from build123d import *

# Parameters (mm, degrees)
SKETCH_2_W          = 16
SKETCH_2_H          = 35
EXTRUDE_1_DEPTH     = 2
EXTRUDE_START       = 1.5
SKETCH_4_R          = 2.6
EXTRUDE_2_DEPTH     = 3
FILLET_2_R          = 1.5
SKETCH_5_R          = 2.1
CUT_EXTRUDE_1_DEPTH = 33.345787979


with BuildPart() as part:
    # 草圖2 → 填料-伸長1 (new body)
    with BuildSketch(Plane(origin=(0, 0, 0), x_dir=(1, 0, 0), z_dir=(0, 1, 0))):
        Rectangle(SKETCH_2_W, SKETCH_2_H)
    extrude(amount=EXTRUDE_1_DEPTH)

    # 草圖4 → 填料-伸長2 (add)
    with BuildSketch(Plane.XY.offset(EXTRUDE_START)):
        with BuildLine():
            Line((8, 20), (8, 2))
            Line((8, 2), (-8, 2))
            Line((-8, 2), (-8, 20))
            ThreePointArc((-8, 20), (0, 28), (8, 20))
        make_face()
        with Locations((0, 20)):
            Circle(SKETCH_4_R, mode=Mode.SUBTRACT)
    extrude_2 = extrude(amount=EXTRUDE_2_DEPTH)

    # 鏡射1: 填料-伸長2 across plane
    add(extrude_2.mirror(Plane.XY))

    # 圓角2
    fillet_2_edges = [part.edges().sort_by_distance(p)[0] for p in [
        (0, 2, 4.5),
        (0, 2, 1.5),
        (0, 2, -4.5),
        (0, 2, -1.5),
    ]]
    fillet(fillet_2_edges, radius=FILLET_2_R - 0.0001)  # a hair under: the kernel refuses the full size

    # 草圖5 → 除料-伸長1 (cut, through all)
    with BuildSketch(Plane(origin=(0, 2, 0), x_dir=(1, 0, 0), z_dir=(0, 1, 0))):
        with Locations(Location((0, -12.5, 0), (0, 0, 270))):
            Circle(SKETCH_5_R)
        with Locations(Location((0, 12.5, 0), (0, 0, 90))):
            Circle(SKETCH_5_R)
    extrude(amount=-CUT_EXTRUDE_1_DEPTH, mode=Mode.SUBTRACT)


solid = part.part
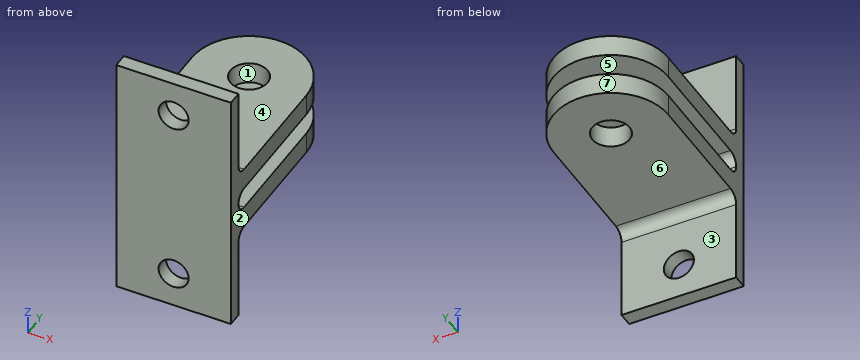
Read the model definition and answer for the solid it produces. Units are mm, in the model's axes. Face numbers are marked on the shaded views. A direction names the side the tool comes from. Coordinates: 2 decimals unless noted, no trailing zeros. Loops run counter-clockwise (first coordinate to the right, second up) from the corner with the lowest first, then second, coordinate; pieces in that order, holes last.
Q1. The part is cut by section B-B on y = 8. Write down the section's boundary in (x, z), and give its area (3 significant figures).
Q2. The part is cut by section C-C on z = -12.5. Write down the section's boundary in (x, y), and give its area (3 significant figures).
Q3. The mould has two halves that part along X. Classify the marked faces 1, 2 and 3: +X half, -X half, draft (parallel to the pull), parting line (faces both ways), or undercut.
Q4. Consider probe 1 along Y at (x, z) = (0, -3.2); probe 2 along Z at (x, y) = (-3, 14.5); probe 3 along X at (y, z) = (0.4, 12.5). Determine where each line is inside the solid, lowest interval first.
Q5. The part is cut by section A-A on x = 0. Give the number of separate pieces and of enclosed holes in the cut face, and give its area (3 significant figures).
Q6. The part is cut by section D-D on y = 21.25. Write down the section's boundary in (x, z).
Q7. Which of the six approach directions +Z, -Z, +X, -X, +Y, -Y give full straight-line access (tool end or side, diameter ignored) to the marked faces 4, 5, 6 and 7?
Q8. Each of these flat-tipped pins is pushed along its axis until it touches: pin 1 Ø3.5 at (x, z) = (3, 14.5) entering from +Y; pin 2 Ø8 at (x, y) = (1, 11) entering from -Z; pin 3 Ø2 at (x, y) = (0.5, 24.5) entering from +Z. Where does it stop, or does it pass through?
Results below:
1. outline: (-8, -4.5) - (8, -4.5) - (8, -1.5) - (-8, -1.5) - close; (-8, 1.5) - (8, 1.5) - (8, 4.5) - (-8, 4.5) - close
1. area: 96.0 mm2
2. outline: (-8, 0) - (-2.1, 0) - (-2.1, 2) - (-8, 2) - close; (2.1, 0) - (8, 0) - (8, 2) - (2.1, 2) - close
2. area: 23.6 mm2
3. face 1: undercut
3. face 2: +X half
3. face 3: draft
4. probe 1: y = 0 to 17.4, 22.6 to 28
4. probe 2: z = -4.5 to -1.5, 1.5 to 4.5
4. probe 3: x = -8 to -2.1, 2.1 to 8
5. separate pieces: 5
5. enclosed holes: 0
5. area: 180 mm2
6. outline: (-7.9, -4.5) - (-2.28, -4.5) - (-2.28, -1.5) - (-7.9, -1.5) - close; (-7.9, 1.5) - (-2.28, 1.5) - (-2.28, 4.5) - (-7.9, 4.5) - close; (2.28, -4.5) - (7.9, -4.5) - (7.9, -1.5) - (2.28, -1.5) - close; (2.28, 1.5) - (7.9, 1.5) - (7.9, 4.5) - (2.28, 4.5) - close
7. face 4: +Z, +X, -X, +Y
7. face 5: +X, -X, +Y
7. face 6: -Z, +X, -X, +Y
7. face 7: +Z, -Z, +Y
8. pin 1: stops at y = 2
8. pin 2: stops at z = -4.5
8. pin 3: stops at z = 4.5
